```python
from build123d import *

# Parameters (mm, degrees)
F1_DEPTH = 574.675
F3_DEPTH = 76.2
F4_R     = 5.08


with BuildPart() as f1:
    # F0 (on Top) → F1 (new body, symmetric)
    with BuildSketch(Plane.XY):
        Polygon((0, 76.2), (0, 0), (76.2, 0), (76.2, 6.35), (6.35, 6.35), (6.35, 76.2), align=None)
    extrude(amount=F1_DEPTH, both=True)

    # F2 (on face) → F3 (cut)
    with BuildSketch(Plane(origin=(0, 0, 0), x_dir=(0, -1, 0), z_dir=(-1, 0, 0))):
        Polygon((-76.2, -574.675), (0, -574.675), (0, -498.475), align=None)
        Polygon((0, 574.675), (-76.2, 574.675), (0, 498.475), align=None)
    extrude(amount=-F3_DEPTH, mode=Mode.SUBTRACT)

    # F4
    f4_edges = [f1.edges().sort_by_distance(p)[0] for p in [
        (6.35, 76.2, 0),
        (6.35, 6.35, 0),
        (76.2, 6.35, 0),
    ]]
    fillet(f4_edges, radius=F4_R)


solid = f1.part
```
Check sheet for the modelled part. Datum: model origin and axes. Units: mm. A direction names the side the tool comes from. Round coordinates to 2 decimals unless told otherwise and drop trailing zeros. Order: outer loops, then holes, each group sorted by start corner. A loop starts at its lowest first (then second) coordinate and runs counter-clockwise, first axis right, second up. Notation, with made-up numbers: M 32.5,-30.5 L 61.5,-30.5 A22 ccw 61.5,2.5 Z; hole C -2.5,-7 d10. An arc over 180 degrees is marked long. Answer in a Markdown table with one row per item.
(1) Section check B-B on x = 36. Record the boundary of the cut face in (y, z) (3 decimals).
Findings:
| item | result |
|---|---|
| outline | M 0,-498.475 L 6.35,-504.825 L 6.35,504.825 L 0,498.475 Z |
(2) Gauge pin test, flat ends, axial feed: pin 1 (18 mm diameter, centred on y = 38.5, z = -233, fed in from +X); pin 2 (3 mm diameter, centred on x = 14.5, z = -222, fed in from +Y); pin 3 (10 mm diameter, centred on x = 10.5, y = 50, fed in from +Z). Record the tip position at first contact, or that the pin passes through.
Findings:
| item | result |
|---|---|
| pin 1 | stops at x = 6.35 |
| pin 2 | stops at y = 6.35 |
| pin 3 | stops at z = 551.26 |
(3) Section check C-C on y = 53. Record the boundary of the cut face in (x, z) (3 decimals).
Findings:
| item | result |
|---|---|
| outline | M 0,-551.475 L 6.35,-551.475 L 6.35,551.475 L 0,551.475 Z |
(4) Set-up check for faces 1 (the flat face through (4.056, 20.989, -519.464)), 2 (the flat face through (6.35, 41, 8)): record each of +Z, -Z, +X, -X, +Y, -Y from which the full face is reachable in a straight line by a thin tool's end or side.
Findings:
| item | result |
|---|---|
| face 1 | -Z, +X, -X, -Y |
| face 2 | +Z, -Z, +X, +Y |
(5) Section check A-A on z = 112. Record the boundary of the cut face in (x, y).
Findings:
| item | result |
|---|---|
| outline | M 0,0 L 76.2,0 L 76.2,1.27 A5.08 ccw 71.12,6.35 L 11.43,6.35 A5.08 cw 6.35,11.43 L 6.35,71.12 A5.08 ccw 1.27,76.2 L 0,76.2 Z |
(6) Material ranges on line 1 along X through (y, z) = (40, -53), recorded low to high. Write a range as from..to.
Findings:
| item | result |
|---|---|
| line 1 | x = 0..6.35 |
